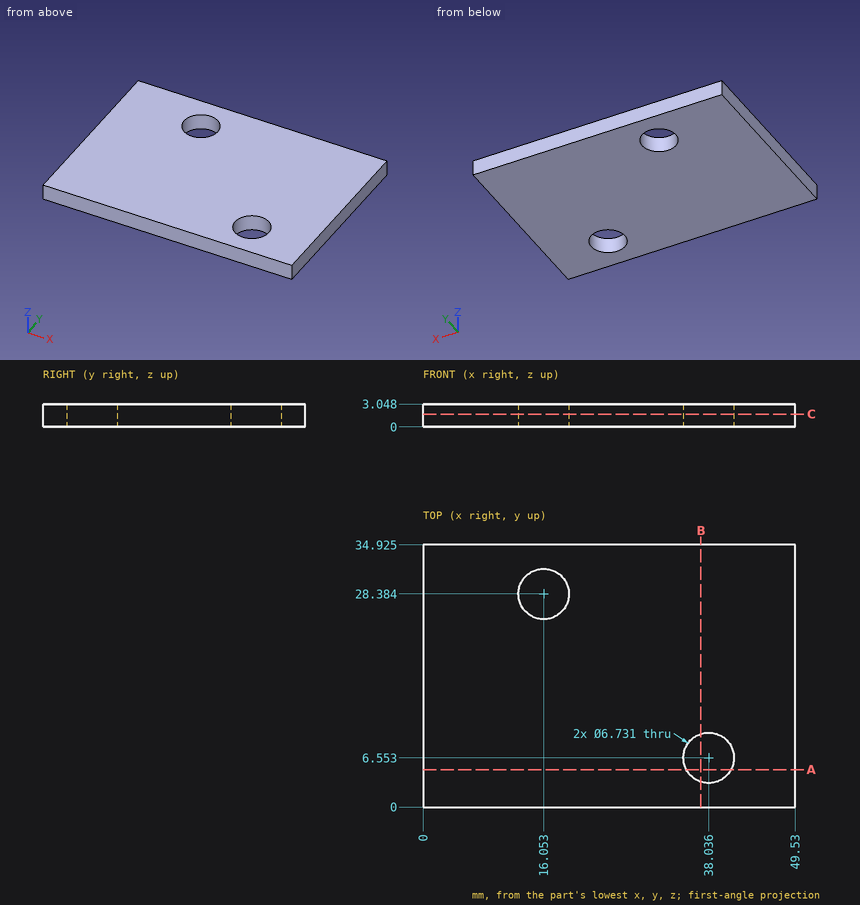
Part print with two shaded views. Sizes in mm from the minimum x, y, z corner. Round coordinates to 2 decimals unless told otherwise and drop trailing zeros. Loops run counter-clockwise (first coordinate to the right, second up) from the corner with the lowest first, then second, coordinate; pieces in that order, holes last. Notation, with made-up numbers: (-37.5, 84.5) - (16.5, 84.5) arc R18 ccw to (16.5, 116.5) - close; hole circle Ø8 at (18.25, 35.5). An arc over 180 degrees is marked (long way). Answer as a JSON object with one key per item and string values.
Item 1: Band-saw the part on B-B on x = 37. List the corners of the cut face in (y, z) (1 decimal).
Output:
{"outline": "(0, 0) - (3.4, 0) - (3.4, 3) - (0, 3) - close; (9.8, 0) - (34.9, 0) - (34.9, 3) - (9.8, 3) - close"}
Item 2: Band-saw the part on A-A on y = 5. List the corners of the cut face in (x, z), plus the area to 3 significant figures.
Output:
{"outline": "(0, 0) - (35.05, 0) - (35.05, 3.05) - (0, 3.05) - close; (41.02, 0) - (49.53, 0) - (49.53, 3.05) - (41.02, 3.05) - close", "area": "133 mm2"}
Item 3: Wall check: L1, parallel to Y at x = 36.5, z = 0.35 (1 decimal); L2, parallel to X at y = 5, z = 2.5; L3, parallel to X at y = 4, z = 1.85 (1 decimal). Give the ranges that are in metal, low to high.
Output:
{"L1": "0 to 3.6, 9.5 to 34.9", "L2": "0 to 35.05, 41.02 to 49.53", "L3": "0 to 35.8, 40.2 to 49.5"}
Item 4: Band-saw the part on C-C on z = 1.7. List the corners of the cut face in (x, y) (1 decimal), plus the area to 3 significant figures.
Output:
{"outline": "(0, 0) - (49.5, 0) - (49.5, 34.9) - (0, 34.9) - close; hole circle Ø6.7 at (16.1, 28.4); hole circle Ø6.7 at (38, 6.6)", "area": "1,660 mm2"}
